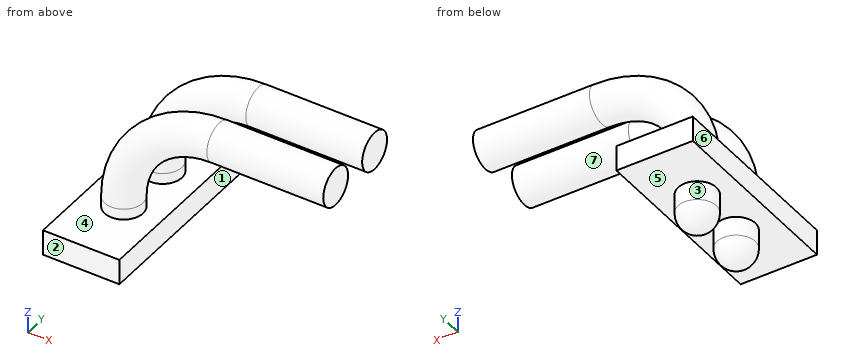
```python
from build123d import *

# Parameters (mm, degrees)
SKETCH1_W           = 6
SKETCH1_H           = 15
BOSS_EXTRUDE1_DEPTH = 2
SKETCH2_R           = 1.5
BOSS_EXTRUDE2_DEPTH = 3
FILLET1_R           = 1.5
SKETCH3_R           = 1.5


with BuildPart() as part:
    # Sketch1 → Boss-Extrude1 (new body)
    with BuildSketch(Plane.XY):
        Rectangle(SKETCH1_W, SKETCH1_H)
    extrude(amount=BOSS_EXTRUDE1_DEPTH)

    # Sketch2 → Boss-Extrude2 (add)
    with BuildSketch(Plane(origin=(0, 0, 0), x_dir=(-1, 0, 0), z_dir=(0, 0, -1))):
        with Locations((0, 2.35)):
            Circle(SKETCH2_R)
        with Locations((0, -2.35)):
            Circle(SKETCH2_R)
    extrude(amount=BOSS_EXTRUDE2_DEPTH)

    # Fillet1
    fillet1_edges = [part.edges().sort_by_distance(p)[0] for p in [
        (1.5, 2.35, -3),
        (1.5, -2.35, -3),
    ]]
    fillet(fillet1_edges, radius=FILLET1_R)

    # Sweep1: sweep along a path in Sketch4
    with BuildLine(Plane(origin=(0, 2.35, 0), x_dir=(-1, 0, 0), z_dir=(0, 1, 0))) as sweep1_path:
        Line((0, 2), (0, 2.85))
        ThreePointArc((0, 2.85), (-2.196699141, 8.153300859), (-7.5, 10.35))
        Line((-7.5, 10.35), (-16.65, 10.35))
    # Sketch3 → Sweep1 (sweep)
    with BuildSketch(Plane.XY.offset(2)):
        with Locations((0, -2.35)):
            Circle(SKETCH3_R)
        with Locations((0, 2.35)):
            Circle(SKETCH3_R)
    sweep(path=sweep1_path.line)


solid = part.part
```
Here's how the part is built. I have some questions about the finished solid (model axes, mm). Face numbers are marked on the shaded views. A direction names the side the tool comes from. Coordinates: 2 decimals unless noted, no trailing zeros. Write each loop counter-clockwise with the first axis right and the second up, starting at its lowest first coordinate (ties: lowest second). Pieces come first, ordered by that corner, then holes. Notation, with made-up numbers: (77.25, -4.5) - (128.25, -4.5) arc R14 ccw to (128.25, 12.5) - close; hole circle Ø11 at (83.5, 24.25). An arc over 180 degrees is marked (long way). One line per item, written item: value.
1) Suppose I cut it at B-B on y = 2.35. Write out the boundary of the cut face in (x, z), and give its area (3 significant figures).
Model answer:
outline: (-3, 0) - (-1.5, 0) - (-1.5, -1.5) arc R1.5 ccw to (1.5, -1.5) - (1.5, 0) - (3, 0) - (3, 2) - (1.5, 2) - (1.5, 2.85) arc R6 cw to (7.5, 8.85) - (16.65, 8.85) - (16.65, 11.85) - (7.5, 11.85) arc R9 ccw to (-1.5, 2.85) - (-1.5, 2) - (-3, 2) - close
area: 85.4 mm²
2) On a 3-axis mill with a long thin cutter (end or side, diameter ignored), from which of +Z, -Z, +X, -X, +Y, -Y can I reach the whole of each face in a straight line? I mean the marked faces 4, 5, 6 and 7. Say none if no direction works.
Model answer:
face 4: none
face 5: -Z
face 6: +Z, -Z, -X, +Y, -Y
face 7: +X
3) Suppose I cut it at C-C on y = -4.5. Write out the boundary of the cut face in (x, z).
Model answer:
outline: (-3, 0) - (3, 0) - (3, 2) - (-3, 2) - close
4) Suppose I cut it at A-A on z = -0.75. Write out the boundary of the cut face in (x, y), and give its area (3 significant figures).
Model answer:
outline: circle Ø3 at (0, -2.35); circle Ø3 at (0, 2.35)
area: 14.1 mm²
5) I need wall thicknesses on line 1 along X through (y, z) = (2, 1.25); line 2 along Y through (x, z) = (1, 8.75); line 3 along Z through (x, y) = (2.5, -6.5). Which ranges of each line are inside material? Lowest first, please.
Model answer:
line 1: x = -3 to 3
line 2: y = -3.13 to -1.57, 1.57 to 3.13
line 3: z = 0 to 2
6) I'm going to push flat-ended pins straight in: P1, Ø1.6, axis at y = 2, z = 1.5, coming from the +X side; P2, Ø4, axis at x = 4.5, y = -4.5, coming from the +Z side; P3, Ø5, axis at x = 11.5, y = 5.5, coming from the -Z side; P4, Ø1, axis at x = 5, z = 5.5, coming from the +Y side. Where does each tip first touch, or does it pass through?
Model answer:
P1: stops at x = 3
P2: stops at z = 11.57
P3: stops at z = 9
P4: passes through
7) We'd pull the mould along Y, two halves only. Please class the marked faces 1, 2 and 3: pulls with the +Y half, pulls with the -Y half, needs draft (parallel to the pull), parting line crosses it, or undercut.
Model answer:
face 1: needs draft
face 2: pulls with the -Y half
face 3: undercut
8) Suppose I cut it at D-D on y = -2. Write out the boundary of the cut face in (x, z).
Model answer:
outline: (-3, 0) - (-1.46, 0) - (-1.46, -1.5) arc R1.46 ccw to (1.46, -1.5) - (1.46, 0) - (3, 0) - (3, 2) - (1.46, 2) - (1.46, 2.85) arc R6.04 cw to (7.5, 8.89) - (16.65, 8.89) - (16.65, 11.81) - (7.5, 11.81) arc R8.96 ccw to (-1.46, 2.85) - (-1.46, 2) - (-3, 2) - close
